```python
from build123d import *

# Parameters (mm, degrees)
SKETCH1_R           = 12.5
SKETCH1_R_2         = 3
BOSS_EXTRUDE1_DEPTH = 15
CHAMFER1_SIZE       = 3
SKETCH2_R           = 6
CUT_EXTRUDE1_DEPTH  = 5


with BuildPart() as part:
    # Sketch1 → Boss-Extrude1 (new body)
    with BuildSketch(Plane(origin=(0, 0, 0), x_dir=(1, 0, 0), z_dir=(0, 1, 0))):
        with Locations(Location((0, 0, 0), (0, 0, 270))):
            Circle(SKETCH1_R)
        with Locations(Location((0, 0, 0), (0, 0, 270))):
            Circle(SKETCH1_R_2, mode=Mode.SUBTRACT)
    extrude(amount=BOSS_EXTRUDE1_DEPTH)

    # Chamfer1
    chamfer1_edges = [part.edges().sort_by_distance(p)[0] for p in [
        (0, 0, -12.5),
    ]]
    chamfer(chamfer1_edges, length=CHAMFER1_SIZE)

    # Sketch2 → Cut-Extrude1 (cut)
    with BuildSketch(Plane.XZ):
        with Locations(Location((0, 0, 0), (0, 0, 270))):
            Circle(SKETCH2_R)
    extrude(amount=-CUT_EXTRUDE1_DEPTH, mode=Mode.SUBTRACT)


solid = part.part
```
Can you work these out from the model? Positions are in its coordinate system, mm. A direction names the side the tool comes from. Coordinates: 2 decimals unless noted, no trailing zeros. Loops run counter-clockwise (first coordinate to the right, second up) from the corner with the lowest first, then second, coordinate; pieces in that order, holes last. Notation, with made-up numbers: (-16.5, 28.25) - (13.5, 28.25) arc R11 cw to (13.5, 37.25) - close; hole circle Ø7 at (-38, 67.5). An arc over 180 degrees is marked (long way). Use a Markdown table: item, result.
Item 1: Will these pins go through, and if not, where does the flat tip stop? pin 1 (8 mm diameter, centred on x = -6.5, y = 6.5, fed in from -Z); pin 2 (6 mm diameter, centred on x = -0.5, z = 1.5, fed in from -Y); pin 3 (3 mm diameter, centred on x = 6, y = 9.5, fed in from +Z).
Numbers:
| item | result |
|---|---|
| pin 1 | stops at z = -12.25 |
| pin 2 | stops at y = 5 |
| pin 3 | stops at z = 11.66 |
Item 2: I want a section at C-C on y = 6. Please give me the cut outline in (x, z), and give its area (3 significant figures).
Numbers:
| item | result |
|---|---|
| outline | circle Ø25 at (0, 0); hole circle Ø6 at (0, 0) |
| area | 463 mm2 |
Item 3: I want a section at B-B on z = 0. Please give me the cut outline in (x, y).
Numbers:
| item | result |
|---|---|
| outline | (-12.5, 3) - (-9.5, 0) - (-6, 0) - (-6, 5) - (-3, 5) - (-3, 15) - (-12.5, 15) - close; (3, 5) - (6, 5) - (6, 0) - (9.5, 0) - (12.5, 3) - (12.5, 15) - (3, 15) - close |
Item 4: If I drill on probe 1 along X at (y, z) = (13.25, 0); probe 2 along Y at (x, z) = (4, -2.5); probe 3 along Z at (x, y) = (0.75, 1.25), over which ranges is the centre line in solid material (lowest first)? Write a range as from..to.
Numbers:
| item | result |
|---|---|
| probe 1 | x = -12.5..-3, 3..12.5 |
| probe 2 | y = 5..15 |
| probe 3 | z = -10.72..-5.95, 5.95..10.72 |
Item 5: We'd pull the mould along X, two halves only. Please class faces 1 (the face through (3.755, 8.916, 11.923)), 2 (the face through (-3, 15, 3)), 3 (the face through (1.802, 2.465, -5.723)): released by +X, released by -X, zero draft, split by the parting line, or undercut.
Numbers:
| item | result |
|---|---|
| face 1 | split by the parting line |
| face 2 | zero draft |
| face 3 | undercut |
Item 6: For faces 4 (the face through (3, 5, -1)), 5 (the face through (0.9, 9.93, 2.86)), which set-ups out of +Z, -Z, +X, -X, +Y, -Y let a thin tool reach every point of the face, with its end or its side?
Numbers:
| item | result |
|---|---|
| face 4 | -Y |
| face 5 | +Y, -Y |
Item 7: I want a section at A-A on x = 0. Please give me the cut outline in (y, z).
Numbers:
| item | result |
|---|---|
| outline | (0, -9.5) - (3, -12.5) - (15, -12.5) - (15, -3) - (5, -3) - (5, -6) - (0, -6) - close; (0, 6) - (5, 6) - (5, 3) - (15, 3) - (15, 12.5) - (3, 12.5) - (0, 9.5) - close |
